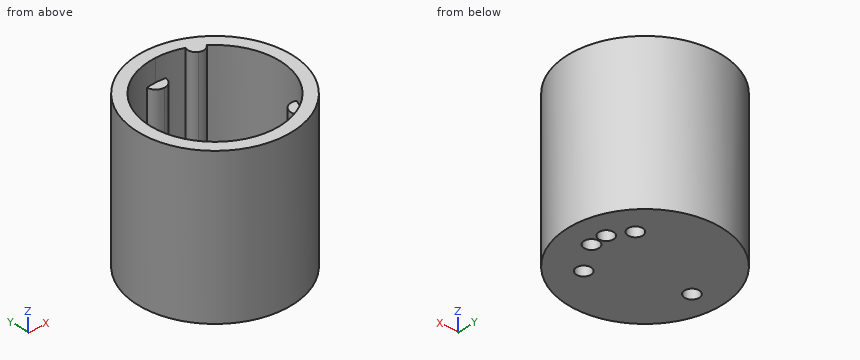
```python
from build123d import *

# Parameters (mm, degrees)
F0_R     = 10.5
F1_DEPTH = 21
F3_DEPTH = 18
F4_R     = 1
F5_DEPTH = 25
F7_DEPTH = 15


with BuildPart() as f1:
    # F0 (on Top) → F1 (new body)
    with BuildSketch(Plane.XY):
        Circle(F0_R)
    extrude(amount=F1_DEPTH)

    # F2 (on face) → F3 (cut)
    with BuildSketch(Plane.XY.offset(21)):
        with BuildLine():
            ThreePointArc((3.875, 6.711697), (3.371846, 7.346729), (3.440033, 8.154059))
            ThreePointArc((3.440033, 8.154059), (1.754862, 8.67427), (0, 8.85))
            Line((0, 8.85), (0, 0))
            Line((0, 0), (3.875, 6.711697))
        make_face()
        with BuildLine():
            Line((0, 0), (0, 8.85))
            ThreePointArc((0, 8.85), (-2.81738, -8.389569), (5.341606, 7.056185))
            ThreePointArc((5.341606, 7.056185), (4.676531, 6.593469), (3.875, 6.711697))
            Line((3.875, 6.711697), (0, 0))
        make_face()
    extrude(amount=-F3_DEPTH, mode=Mode.SUBTRACT)

    # F4 (on face) → F5 (cut)
    with BuildSketch(Plane.XY.offset(3)):
        with Locations((-6.9, -0.5)):
            Circle(F4_R)
        with Locations((5, 4)):
            Circle(F4_R)
        with Locations((6.7, 1.5)):
            Circle(F4_R)
        with Locations((4, -4.8)):
            Circle(F4_R)
        with Locations((6.7, -0.7)):
            Circle(F4_R)
    extrude(amount=-F5_DEPTH, mode=Mode.SUBTRACT)

    # F6 (on face) → F7 (join)
    with BuildSketch(Plane.XY.offset(3)):
        with BuildLine():
            ThreePointArc((0, 7.55), (0.919239, 7.930761), (1.3, 8.85))
            ThreePointArc((1.3, 8.85), (-0.919239, 9.769239), (0, 7.55))
        make_face()
        with BuildLine():
            ThreePointArc((8.964325, -4.425), (8.00079, -3.169296), (6.538492, -3.775))
            ThreePointArc((6.538492, -3.775), (7.32786, -5.680704), (8.964325, -4.425))
        make_face()
        with BuildLine():
            ThreePointArc((-6.364325, -4.425), (-6.408621, -4.088535), (-6.538492, -3.775))
            ThreePointArc((-6.538492, -3.775), (-8.920028, -4.761465), (-6.364325, -4.425))
        make_face()
    extrude(amount=F7_DEPTH)


solid = f1.part
```
CAD build for the part. Positions are in the model's coordinates, mm. Round coordinates to 2 decimals unless told otherwise and drop trailing zeros. Write each loop counter-clockwise with the first axis right and the second up, starting at its lowest first coordinate (ties: lowest second). Pieces come first, ordered by that corner, then holes.
Item 1: Drop flat-ended pins along their axis: pin 1 Ø2 at (y, z) = (-2, 15.5) entering from +X; pin 2 Ø3 at (x, y) = (5, 4) entering from +Z; pin 3 Ø1.4 at (x, y) = (0, 8) entering from +Z. Give the stop position or say it passes through.
Filled in:
pin 1: stops at x = 10.45
pin 2: stops at z = 3
pin 3: stops at z = 18
Item 2: Drill centre lines: L1, parallel to Y at x = -6.75, z = 11.25; L2, parallel to Y at x = 6.7, z = 0.7; L3, parallel to X at y = 0.25, z = 19.5. Where is each one in solid material? Low to high.
Filled in:
L1: y = -8.04 to -5.72, -5.35 to -3.5, 5.72 to 8.04
L2: y = -8.08 to -1.7, 0.3 to 0.5, 2.5 to 8.08
L3: x = -10.5 to -8.85, 8.85 to 10.5
Item 3: Band-saw the part on A-A on y = 4. Write the cut outline in (x, z), then the cut area to 3 significant figures.
Filled in:
outline: (-9.71, 0) - (4, 0) - (4, 3) - (-7.89, 3) - (-7.89, 21) - (-9.71, 21) - close; (6, 0) - (9.71, 0) - (9.71, 21) - (7.89, 21) - (7.89, 3) - (6, 3) - close
area: 118 mm2
Item 4: Band-saw the part on D-D on x = -4.5. Write the cut outline in (y, z), then the cut area to 3 significant figures.
Filled in:
outline: (-9.49, 0) - (9.49, 0) - (9.49, 21) - (7.62, 21) - (7.62, 3) - (-7.62, 3) - (-7.62, 21) - (-9.49, 21) - close
area: 124 mm2
Item 5: Band-saw the part on C-C on y = 0. Write the cut outline in (x, z), then the cut area to 3 significant figures.
Filled in:
outline: (-10.5, 0) - (-7.77, 0) - (-7.77, 3) - (-8.85, 3) - (-8.85, 21) - (-10.5, 21) - close; (-6.03, 0) - (5.99, 0) - (5.99, 3) - (-6.03, 3) - close; (7.41, 0) - (10.5, 0) - (10.5, 21) - (8.85, 21) - (8.85, 3) - (7.41, 3) - close
area: 113 mm2
